CAD build for the part. Positions are in the model's coordinates, mm. Face numbers are marked on the shaded views. A direction names the side the tool comes from. Coordinates: 2 decimals unless noted, no trailing zeros. Loops run counter-clockwise (first coordinate to the right, second up) from the corner with the lowest first, then second, coordinate; pieces in that order, holes last. Notation, with made-up numbers: (3, 2.5) -> (37, 2.5) arc R23 ccw to (37, 25.5) -> close; hole circle Ø1 at (-5.5, 40). An arc over 180 degrees is marked (long way). Write each question's results on one line, items separated by ' | '.
from build123d import *

# Parameters (mm, degrees)
F0_R     = 50
F1_DEPTH = 300


with BuildPart() as f1:
    # F0 (on Front) → F1 (new body)
    with BuildSketch(Plane.XZ):
        Polygon((-150, -150), (-300, 0), (-388.388348, -88.388348), (-147.972042, -328.804653), (-121.47121, -302.303821), (-86.084527, -266.917138), (-59.583694, -240.416306), align=None)
        Polygon((-374.246212, -88.388348), (-300, -14.142136), (-73.72583, -240.416306), (-147.972042, -314.662518), align=None, mode=Mode.SUBTRACT)
        Polygon((-150, 150), (-300, 0), (-150, -150), (0, 0), (150, -150), (225.000005, -74.999995), (300, 0), (150, 150), align=None)
        Polygon((0, 14.142136), (-150, -135.857864), (-285.857864, 0), (-145.857864, 140), (145.857864, 140), (285.857864, 0), (217.928937, -67.928927), (150, -135.857864), align=None, mode=Mode.SUBTRACT)
        Polygon((388.388348, -88.388348), (300, 0), (225.000005, -74.999995), (150, -150), (59.583694, -240.416306), (86.084527, -266.917138), (121.47121, -302.303821), (147.972042, -328.804653), align=None)
        Polygon((147.972042, -314.662518), (73.72583, -240.416306), (300, -14.142136), (374.246212, -88.388348), align=None, mode=Mode.SUBTRACT)
        with BuildLine():
            Line((-86.084527, -266.917138), (-121.47121, -302.303821))
            Line((-121.47121, -302.303821), (-57.075043, -361.494856))
            ThreePointArc((-57.075043, -361.494856), (-44.174127, -339.39646), (-23.238764, -324.683088))
            Line((-23.238764, -324.683088), (-86.084527, -266.917138))
        make_face()
        with BuildLine():
            ThreePointArc((-23.238764, -324.683088), (-44.174127, -339.39646), (-57.075043, -361.494856))
            ThreePointArc((-57.075043, -361.494856), (-9.367444, -439.264243), (59.999994, -379.999995))
            ThreePointArc((59.999994, -379.999995), (59.264243, -370.632559), (57.075032, -361.494859))
            ThreePointArc((57.075032, -361.494859), (44.174118, -339.396463), (23.238756, -324.68309))
            ThreePointArc((23.238756, -324.68309), (-4e-06, -319.999995), (-23.238764, -324.683088))
        make_face()
        with Locations((-6e-06, -379.999995)):
            Circle(F0_R, mode=Mode.SUBTRACT)
        with BuildLine():
            Line((121.47121, -302.303821), (86.084527, -266.917138))
            Line((86.084527, -266.917138), (23.238756, -324.68309))
            ThreePointArc((23.238756, -324.68309), (44.174118, -339.396463), (57.075032, -361.494859))
            Line((57.075032, -361.494859), (121.47121, -302.303821))
        make_face()
        Polygon((0, 0), (-150, -150), (-59.583694, -240.416306), (0, -300), (59.583694, -240.416306), (150, -150), align=None)
        Polygon((125.857864, -160), (0, -285.857864), (-125.857864, -160), (-135.857864, -150), (-67.928932, -82.071068), (0, -14.142136), (67.928932, -82.071068), (135.857864, -150), align=None, mode=Mode.SUBTRACT)
        Polygon((-135.857864, -150), (-125.857864, -160), (125.857864, -160), (135.857864, -150), align=None)
    extrude(amount=F1_DEPTH)


solid = f1.part
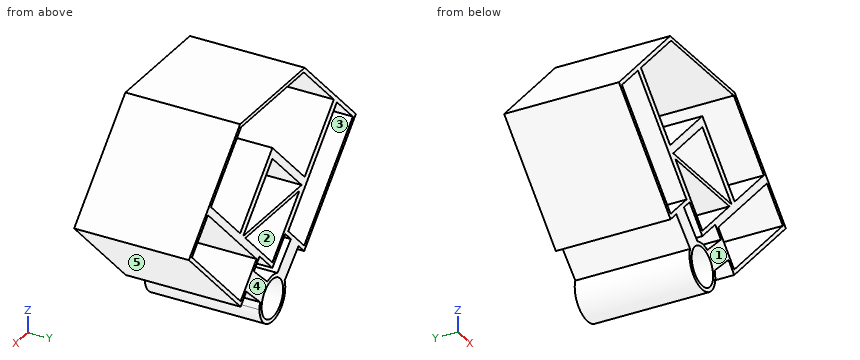
1) Slice it at C-C (z = 45). Write the cut outline in (x, y).
Outcome:
outline: (-255, -300) -> (-240.86, -300) -> (-240.86, 0) -> (-255, 0) -> close; (240.86, -300) -> (255, -300) -> (255, 0) -> (240.86, 0) -> close
2) Slice it at D-D (x = 318.5). Write the cut outline in (y, z), then the cut area to 3 significant figures.
Outcome:
outline: (-300, -158.28) -> (0, -158.28) -> (0, -144.13) -> (-300, -144.13) -> close; (-300, -32.64) -> (0, -32.64) -> (0, -18.5) -> (-300, -18.5) -> close | area: 8,490 mm^2
3) Slice it at A-A (z = -42). Write the cut outline in (x, y), then the cut area to 3 significant figures.
Outcome:
outline: (-342, -300) -> (-327.86, -300) -> (-327.86, 0) -> (-342, 0) -> close; (-272.14, -300) -> (-243.86, -300) -> (-243.86, 0) -> (-272.14, 0) -> close; (-56.14, -300) -> (-27.86, -300) -> (-27.86, 0) -> (-56.14, 0) -> close; (27.86, -300) -> (56.14, -300) -> (56.14, 0) -> (27.86, 0) -> close; (243.86, -300) -> (272.14, -300) -> (272.14, 0) -> (243.86, 0) -> close; (327.86, -300) -> (342, -300) -> (342, 0) -> (327.86, 0) -> close | area: 42,400 mm^2
4) Pin check, flat tips, straight feed: pin 1 (8 mm diameter, centred on x = 212, y = -107.5, fed in from +Z); pin 2 (10 mm diameter, centred on x = -43, z = -147, fed in from +Y); pin 3 (3 mm diameter, centred on y = -199, z = -185.5, fed in from -X); pin 4 (3 mm diameter, centred on x = 162.5, y = -219, fed in from -Z). Stop position of each tip, or through.
Outcome:
pin 1: stops at z = 92 | pin 2: stops at y = 0 | pin 3: stops at x = -292.78 | pin 4: stops at z = -315.78
5) Drill centre lines: L1, parallel to Z at x = -32.5, y = -195.5; L2, parallel to Z at x = -22, y = -99; L3, parallel to X at y = -109, z = -146. Where is each one in solid material? Low to high. Write a range as from..to.
Outcome:
L1: z = -430.44..-418, -342..-316.17, -267.5..-253.36, -160..-150, -46.64..-18.36, 140..150 | L2: z = -435.82..-424.9, -335.1..-324.18, -278..-263.86, -160..-150, -36.14..-7.86, 140..150 | L3: x = -330.78..-316.63, -168.14..-131.86, 131.86..168.14, 316.63..330.78
6) Which spindle directions (+Z, -Z, +X, -X, +Y, -Y) get a long thin tool onto all of the face, cutting with end or side? Do the marked faces 1 and 2. Say none if no direction does.
Outcome:
face 1: +Z, -Z, +X, -X, -Y | face 2: +Y, -Y
7) Slice it at B-B (x = -13). Write the cut outline in (y, z).
Outcome:
outline: (-300, -438.57) -> (0, -438.57) -> (0, -428.28) -> (-300, -428.28) -> close; (-300, -331.72) -> (0, -331.72) -> (0, -321.43) -> (-300, -321.43) -> close; (-300, -287) -> (0, -287) -> (0, -272.86) -> (-300, -272.86) -> close; (-300, -160) -> (0, -160) -> (0, -150) -> (-300, -150) -> close; (-300, -27.14) -> (0, -27.14) -> (0, 1.14) -> (-300, 1.14) -> close; (-300, 140) -> (0, 140) -> (0, 150) -> (-300, 150) -> close
8) Two-plate mould, pull along Z, no slides. Class the marked faces 3, 4 and 5: pulls with the +Z half, pulls with the -Z half, needs draft (parallel to the pull), parting line crosses it, or undercut.
Outcome:
face 3: undercut | face 4: needs draft | face 5: pulls with the -Z half
